```python
from build123d import *

# Parameters (mm, degrees)
F0_W         = 160
F0_H         = 120
F0_W_2       = 140
F0_H_2       = 100
F1_DEPTH     = 153.4
F2_W         = 160
F2_H         = 120
F3_DEPTH     = 25
F5_W         = 3
F5_H         = 25
F5_W_2       = 2.5065724061
F5_H_2       = 21.7677888939
F7_W         = 10.3015974164
F7_H         = 119.727473706
F8_DEPTH     = 160
F9_R         = 10.5745800983
F10_DEPTH    = 5
F11_W        = 7
F11_H        = 7
F12_DEPTH    = 21.1
F13_R        = 2.005862126
F14_DEPTH    = 20
F15_R        = 2.1
F16_DEPTH    = 20
F17_R        = 2.1
F18_DEPTH    = 20
F19_R        = 2.218699255
F20_DEPTH    = 20
F21_W        = 45
F21_H        = 30
F22_DEPTH    = 5
F23_W        = 35
F23_H        = 7.2088057839
F24_DEPTH    = 5
F25_W        = 8
F25_H        = 3.5
F26_DEPTH    = 5
F27_W        = 140
F27_H        = 4.4944308201
F28_DEPTH    = 176
F29_W        = 29
F29_H        = 3.2
F30_DEPTH    = 5
F31_R        = 5
F32_T1_DEPTH = 185
F32_T3_DEPTH = 144.727473706
F32_T5_DEPTH = 172.5


# Not quite as in the source:
# - a fillet or chamfer that OpenCascade refuses, or shapes differently, is made with other operations: its cross-section is extruded or revolved along the edge and cut away or added


with BuildPart() as f1:
    # F0 (on Front) → F1 (new body)
    with BuildSketch(Plane.XZ):
        Rectangle(F0_W, F0_H)
        Rectangle(F0_W_2, F0_H_2, mode=Mode.SUBTRACT)
    extrude(amount=-F1_DEPTH)

    # F2 (on face) → F3 (join)
    with BuildSketch(Plane(origin=(0, 153.4, 0), x_dir=(-1, 0, 0), z_dir=(0, 1, 0))):
        Rectangle(F2_W, F2_H)
    extrude(amount=F3_DEPTH)

    # F5 (on face) → F6 (revolve)
    with BuildSketch(Plane.XZ):
        with Locations((-75.5, 22.5)):
            Rectangle(F5_W, F5_H)
        with Locations((-75.746713797, -24.116105553)):
            Rectangle(F5_W_2, F5_H_2)
    revolve(axis=Axis((-74, 0, 22.5), (0, 0, -1)))

    # F7 (on face) → F8 (join)
    with BuildSketch(Plane.XZ):
        with Locations((-75.0872157514, 0.2289246768)):
            Rectangle(F7_W, F7_H)
    extrude(amount=F8_DEPTH)

    # F9 (on face) → F10 (join)
    with BuildSketch(Plane(origin=(-80.2380144596, 0, 0), x_dir=(0, -1, 0), z_dir=(-1, 0, 0))):
        with Locations((78.2749652863, 0)):
            Circle(F9_R)
    extrude(amount=F10_DEPTH)

    # F11 (on face) → F12 (join)
    with BuildSketch(Plane(origin=(-85.2380144596, 0, 0), x_dir=(0, -1, 0), z_dir=(-1, 0, 0))):
        with Locations((78.2749652863, 0)):
            Rectangle(F11_W, F11_H)
    extrude(amount=F12_DEPTH)

    # F13 (on face) → F14 (join)
    with BuildSketch(Plane.XY.offset(3.5)):
        with Locations((-102.9334535655, -78.1808274122)):
            Circle(F13_R)
    extrude(amount=F14_DEPTH)

    # F15 (on face) → F16 (join)
    with BuildSketch(Plane(origin=(0, -74.7749652863, 0), x_dir=(-1, 0, 0), z_dir=(0, 1, 0))):
        with Locations((102.8380144596, 0)):
            Circle(F15_R)
    extrude(amount=F16_DEPTH)

    # F17 (on face) → F18 (join)
    with BuildSketch(Plane.XZ.offset(81.7749652863)):
        with Locations((-102.8380144596, 0)):
            Circle(F17_R)
    extrude(amount=F18_DEPTH)

    # F19 (on face) → F20 (join)
    with BuildSketch(Plane(origin=(0, 0, -3.5), x_dir=(1, 0, 0), z_dir=(0, 0, -1))):
        with Locations((-102.7212624934, 78.1562660312)):
            Circle(F19_R)
    extrude(amount=F20_DEPTH)

    # F21 (on face) → F22 (join)
    with BuildSketch(Plane(origin=(-80.2380144596, 0, 0), x_dir=(0, -1, 0), z_dir=(-1, 0, 0))):
        with Locations((32.2962999344, 34.3826470941)):
            Rectangle(F21_W, F21_H)
    extrude(amount=F22_DEPTH)

    # F23 (on face) → F24 (cut)
    with BuildSketch(Plane(origin=(-85.2380144596, 0, 0), x_dir=(0, -1, 0), z_dir=(-1, 0, 0))):
        with Locations((32.0492885076, 42.2782442022)):
            Rectangle(F23_W, F23_H)
    extrude(amount=-F24_DEPTH, mode=Mode.SUBTRACT)

    # F25 (on face) → F26 (join)
    with BuildSketch(Plane(origin=(-85.2380144596, 0, 0), x_dir=(0, -1, 0), z_dir=(-1, 0, 0))):
        with Locations((21.2962999344, 33.4238413102)):
            Rectangle(F25_W, F25_H)
        with Locations((31.7962999344, 33.4238413102)):
            Rectangle(F25_W, F25_H)
        with Locations((42.2962999344, 33.4238413102)):
            Rectangle(F25_W, F25_H)
        with Locations((21.2962999344, 27.9238413102)):
            Rectangle(F25_W, F25_H)
        with Locations((31.7962999344, 27.9238413102)):
            Rectangle(F25_W, F25_H)
        with Locations((42.2962999344, 27.9238413102)):
            Rectangle(F25_W, F25_H)
    extrude(amount=F26_DEPTH)

    # F27 (on face) → F28 (join)
    with BuildSketch(Plane.XZ):
        with Locations((-0.2423568684, -2.24721541)):
            Rectangle(F27_W, F27_H)
    extrude(amount=-F28_DEPTH)

    # F29 (on face) → F30 (join)
    with BuildSketch(Plane(origin=(-85.2380144596, 0, 0), x_dir=(0, -1, 0), z_dir=(-1, 0, 0))):
        with Locations((31.9544213465, 23.1566587463)):
            Rectangle(F29_W, F29_H)
    extrude(amount=F30_DEPTH)

    # F31
    f31_edges = [f1.edges().sort_by_distance(p)[0] for p in [
        (-80, 89.2, 60),
        (0, 178.4, 60),
        (80, 89.2, 60),
        (80, 178.4, 0),
        (-80, 178.4, 0),
    ]]
    fillet(f31_edges, radius=F31_R)

    # F32: fillet of radius 5 on 3 edges, made by hand

    # F32_s2 → F32_t1 (cut)
    with BuildSketch(Plane.XZ.offset(-12.5)):
        with BuildLine():
            ThreePointArc((-75.2380144596, 60.0926615298), (-78.7735483655, 58.6281954357), (-80.2380144596, 55.0926615298))
            Line((-80.2380144596, 55.0926615298), (-80.2380144596, 60.0926615298))
            Line((-80.2380144596, 60.0926615298), (-75.2380144596, 60.0926615298))
        make_face()
    extrude(amount=F32_T1_DEPTH, mode=Mode.SUBTRACT)

    # F32_s4 → F32_t3 (cut)
    with BuildSketch(Plane.XY.offset(-72.1348121762)):
        with BuildLine():
            ThreePointArc((-80.2380144596, -155), (-78.7735483655, -158.5355339059), (-75.2380144596, -160))
            Line((-75.2380144596, -160), (-80.2380144596, -160))
            Line((-80.2380144596, -160), (-80.2380144596, -155))
        make_face()
    extrude(amount=F32_T3_DEPTH, mode=Mode.SUBTRACT)

    # F32_s6 → F32_t5 (cut)
    with BuildSketch(Plane.XZ):
        with BuildLine():
            ThreePointArc((-75.2380144596, -59.6348121762), (-78.7735483655, -58.1703460822), (-80.2380144596, -54.6348121762))
            Line((-80.2380144596, -54.6348121762), (-80.2380144596, -59.6348121762))
            Line((-80.2380144596, -59.6348121762), (-75.2380144596, -59.6348121762))
        make_face()
    extrude(amount=F32_T5_DEPTH, mode=Mode.SUBTRACT)


solid = f1.part
```
Here's how the part is built. I have some questions about the finished solid (model axes, mm). A direction names the side the tool comes from. Coordinates: 2 decimals unless noted, no trailing zeros. Write each loop counter-clockwise with the first axis right and the second up, starting at its lowest first coordinate (ties: lowest second). Pieces come first, ordered by that corner, then holes. Notation, with made-up numbers: M 44,10.25 L 60,10.25 A13 cw 60,31.25 Z; hole C 52.25,-22.5 d4. An arc over 180 degrees is marked long. Answer as CSV lines item,"result". Start each with the question number.
Q1. Will these pins go through, and if not, where does the flat tip stop? pin 1 Ø1.3 at (x, z) = (-103.5, 0.5) entering from -Y; pin 2 Ø1.8 at (y, z) = (-43, 33.5) entering from -X; pin 3 Ø2 at (x, z) = (-83.5, 44) entering from -Y; pin 4 Ø10.5 at (y, z) = (-82, 2.5) entering from -X.
Q2. Suppose I cut it at B-B, the plane y = 52.5. List the corners of the cut face in (x, z) for me.
Q3. Suppose I cut it at D-D, the plane x = 50. List the corners of the cut face in (y, z) for me.
Q4. I need wall thicknesses on probe 1 along Z at (x, y) = (58, 43.5); probe 2 along X at (y, z) = (73, -31); probe 3 along Y at (x, z) = (-65, 17). Which ranges of each line are inside material? Lowest first, please. Write a range as [from, to].
Q5. If we mould it in two halves opening along Z, with no side actions, what happens to faces 4 (the flat face through (-96, -81.775, 0)), 5 (the flat face through (-1, 76, -50)), 6 (the cylindrical face through (-82.703, -88.043, -4.05))? For each: pulls with the +Z half, pulls with the -Z half, needs draft (parallel to the pull), parting line crosses it, or undercut.
Q6. Suppose I cut it at C-C, the plane z = -36.5. List the corners of the cut face in (x, y) for me, then the cut area to 3 significant figures.
Q7. For faces 1 (the flat face through (-80, 85, -3)), 2 (the flat face through (-85.238, -78, -5)), 3 (the flat face through (-69.936, -79, -1)), which set-ups out of +Z, -Z, +X, -X, +Y, -Y let a thin tool reach every point of the face, with its end or its side?
Q8. Suppose I cut it at A-A, the plane y = -93. List the corners of the cut face in (x, z) for me.
Entries:
1,pin 1,"stops at y = -101.77"
1,pin 2,"stops at x = -90.24"
1,pin 3,"stops at y = -54.8"
1,pin 4,"stops at x = -106.34"
2,outline,"M -80,-60 L 80,-60 L 80,55 A5 ccw 75,60 L -75,60 A5 ccw -80,55 Z; hole M -70,-50 L 70,-50 L 70,50 L -70,50 L -70,0 L 69.76,0 L 69.76,-4.49 L -70,-4.49 Z"
3,outline,"M 0,-60 L 178.4,-60 L 178.4,55 A5 ccw 173.4,60 L 0,60 L 0,50 L 153.4,50 L 153.4,0 L 0,0 L 0,-4.49 L 153.4,-4.49 L 153.4,-50 L 0,-50 Z"
4,probe 1,"z = [-60, -50], [-4.49, 0], [50, 60]"
4,probe 2,"x = [-80, -70], [70, 80]"
4,probe 3,"y = [153.4, 178.4]"
5,face 4,"needs draft"
5,face 5,"undercut"
5,face 6,"parting line crosses it"
6,outline,"M -80.24,-155 A5 ccw -75.24,-160 L -69.94,-160 L -69.94,0 L -70,0 L -70,153.4 L 70,153.4 L 70,0 L 80,0 L 80,173.4 A5 ccw 75,178.4 L -75,178.4 A5 ccw -80,173.4 L -80,0 L -80.24,0 Z"
6,area,"8,700 mm²"
7,face 1,"+Z, -Z, -X, +Y"
7,face 2,"none"
7,face 3,"+Z, -Z, +X, -Y"
8,outline,"C -102.84,0 d4.2; M -80.24,-54.63 A5 ccw -75.24,-59.63 L -69.94,-59.63 L -69.94,60.09 L -75.24,60.09 A5 ccw -80.24,55.09 Z"
